Here's how the part is built. I have some questions about the finished solid (model axes, mm). Face numbers are marked on the shaded views. A direction names the side the tool comes from. Round coordinates to 2 decimals unless told otherwise and drop trailing zeros. Loops run counter-clockwise (first coordinate to the right, second up) from the corner with the lowest first, then second, coordinate; pieces in that order, holes last. Notation, with made-up numbers: M 47,-9.5 L 60,-9.5 A7 ccw 60,-3.5 Z; hole C -35.75,-33 d9. An arc over 180 degrees is marked long. Answer as CSV lines item,"result".
```python
from build123d import *

# Parameters (mm, degrees)
F0_R     = 13
F0_R_2   = 2.5
F1_DEPTH = 2.5
F2_R     = 13.5
F2_R_2   = 10.9075922355
F3_DEPTH = 0.8
F4_R     = 13.5
F4_R_2   = 11.2490689916
F5_DEPTH = 0.8
F6_R     = 4
F6_R_2   = 2.5
F7_DEPTH = 2
F7_TAPER = -20


# Not quite as in the source:
# - a fillet or chamfer that OpenCascade refuses, or shapes differently, is made with other operations: its cross-section is extruded or revolved along the edge and cut away or added


with BuildPart() as f1:
    # F0 (on Front) → F1 (new body)
    with BuildSketch(Plane.XZ):
        Circle(F0_R)
        with BuildLine():
            ThreePointArc((-1.7385059182, -10.6337636412), (-7.9358324082, -7.2884769323), (-10.7429600727, -0.8295425725))
            Line((-10.7429600727, -0.8295425725), (-3.9130370712, -0.8295425725))
            ThreePointArc((-3.9130370712, -0.8295425725), (-3.1475751054, -2.468353896), (-1.7385059182, -3.6024432227))
            Line((-1.7385059182, -3.6024432227), (-1.7385059182, -10.6337636412))
        make_face(mode=Mode.SUBTRACT)
        with BuildLine():
            Line((3.9130370712, -0.8295425725), (10.7429600727, -0.8295425725))
            ThreePointArc((10.7429600727, -0.8295425725), (7.9358324082, -7.2884769323), (1.7385059182, -10.6337636412))
            Line((1.7385059182, -10.6337636412), (1.7385059182, -3.6024432227))
            ThreePointArc((1.7385059182, -3.6024432227), (3.1475751054, -2.468353896), (3.9130370712, -0.8295425725))
        make_face(mode=Mode.SUBTRACT)
        with BuildLine():
            ThreePointArc((-1.7385059182, 3.6024432227), (-3.1475751054, 2.468353896), (-3.9130370712, 0.8295425725))
            Line((-3.9130370712, 0.8295425725), (-10.7429600727, 0.8295425725))
            ThreePointArc((-10.7429600727, 0.8295425725), (-7.9358324082, 7.2884769323), (-1.7385059182, 10.6337636412))
            Line((-1.7385059182, 10.6337636412), (-1.7385059182, 3.6024432227))
        make_face(mode=Mode.SUBTRACT)
        Circle(F0_R_2, mode=Mode.SUBTRACT)
        with BuildLine():
            ThreePointArc((1.7385059182, 10.6337636412), (7.9358324082, 7.2884769323), (10.7429600727, 0.8295425725))
            Line((10.7429600727, 0.8295425725), (3.9130370712, 0.8295425725))
            ThreePointArc((3.9130370712, 0.8295425725), (3.1475751054, 2.468353896), (1.7385059182, 3.6024432227))
            Line((1.7385059182, 3.6024432227), (1.7385059182, 10.6337636412))
        make_face(mode=Mode.SUBTRACT)
    extrude(amount=F1_DEPTH)

    # F2 (on face) → F3 (join)
    with BuildSketch(Plane(origin=(0, 0, 0), x_dir=(-1, 0, 0), z_dir=(0, 1, 0))):
        Circle(F2_R)
        Circle(F2_R_2, mode=Mode.SUBTRACT)
    extrude(amount=-F3_DEPTH)

    # F4 (on face) → F5 (join)
    with BuildSketch(Plane.XZ.offset(2.5)):
        Circle(F4_R)
        Circle(F4_R_2, mode=Mode.SUBTRACT)
    extrude(amount=-F5_DEPTH)

    # F6 (on face) → F7 (join)
    with BuildSketch(Plane(origin=(0, 0, 0), x_dir=(-1, 0, 0), z_dir=(0, 1, 0))):
        Circle(F6_R)
        Circle(F6_R_2, mode=Mode.SUBTRACT)
    extrude(amount=F7_DEPTH, taper=F7_TAPER)

    # F8: chamfer of 0.4 on 4 edges, made by hand

    # F8_s1 → F8_t2 (revolve, cut)
    with BuildSketch(Plane.XY):
        Polygon((13.5, -2.1), (13.1, -1.7), (13.5, -1.7), align=None)
    revolve(axis=Axis((0, -1.7, 0), (0, -1, 0)), mode=Mode.SUBTRACT)

    # F8_s3 → F8_t4 (revolve, cut)
    with BuildSketch(Plane.XY):
        Polygon((-13.5, -0.4), (-13.1, -0.8), (-13.5, -0.8), align=None)
    revolve(axis=Axis((0, -0.8, 0), (0, 1, 0)), mode=Mode.SUBTRACT)

    # F8_s5 → F8_t6 (revolve, cut)
    with BuildSketch(Plane.XY):
        Polygon((2.9, -2.5), (2.5, -2.1), (2.5, -2.5), align=None)
    revolve(axis=Axis((0, -2.5, 0), (0, -1, 0)), mode=Mode.SUBTRACT)

    # F8_s7 → F8_t8 (revolve, cut)
    with BuildSketch(Plane.XY):
        Polygon((-4.5325583141, 1.4631919427), (-4.1566812658, 2), (-4.7279404685, 2), align=None)
    revolve(axis=Axis((0, 2, 0), (0, -1, 0)), mode=Mode.SUBTRACT)


solid = f1.part
```
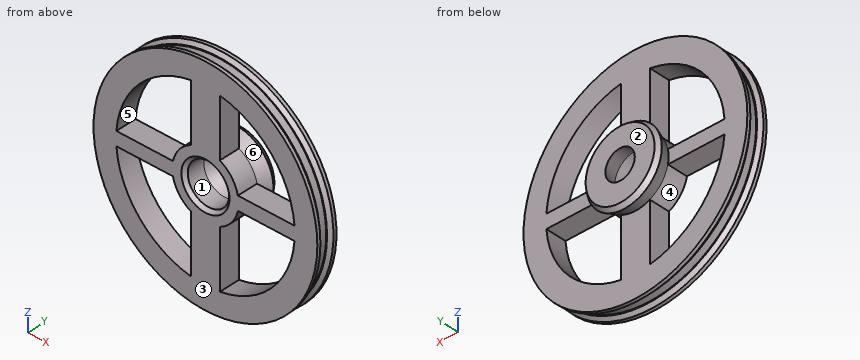
1. I want a section at A-A, the plane x = 7.75. Count the separate pieces of the cut face and the enclosed holes in it, and give its area (3 significant figures).
Evaluation:
separate pieces,"3"
enclosed holes,"0"
area,"20.5 mm²"
2. For P1, Ø2, axis at x = -8, y = -1, coming from the -Z side; P2, Ø1.5, axis at y = 1.5, z = -3, coming from the +X side; P3, Ø1.2, axis at x = 8, y = -1.5, coming from the -Z side; P4, Ø1, axis at y = 1, z = 10.5, coming from the +X side, each with a flat end and sliding along its axis, tell me the tip position at first contact or that it passes through.
Evaluation:
P1,"stops at z = -11.42"
P2,"stops at x = 3.93"
P3,"stops at z = -10.99"
P4,"passes through"
3. I want a section at B-B, the plane y = 0.6. Please give me the cut outline in (x, z).
Evaluation:
outline,"C 0,0 d8.44; hole C 0,0 d4.56"
4. Which directions (+Z, -Z, +X, -X, +Y, -Y) give clear straight access to the entire face, cutting with the end or side of a thin tool? Please do the marked faces 3, 4, 5 and 6.
Evaluation:
face 3,"+Z, -Z, +X, -X, -Y"
face 4,"-Y"
face 5,"+Y, -Y"
face 6,"none"
5. We'd pull the mould along X, two halves only. Please class the marked faces 1 and 2: pulls with the +X half, pulls with the -X half, needs draft (parallel to the pull), parting line crosses it, or undercut.
Evaluation:
face 1,"undercut"
face 2,"needs draft"
6. If I drill on line 1 (Z direction, x = 3.5, y = -1.35); line 2 (Z direction, x = -3, y = -1.25); line 3 (X direction, y = -1.6, z = 0), over which ranges is the centre line in solid material (lowest first)? Write a range as [from, to].
Evaluation:
line 1,"z = [-12.52, -10.19], [-1.94, 1.94], [10.19, 12.52]"
line 2,"z = [-12.65, -10.35], [-2.65, 2.65], [10.35, 12.65]"
line 3,"x = [-13, -2.5], [2.5, 13]"
